Part model, mm, in its own coordinate system. Give positions to 0.01 mm unless a question says otherwise; leave off trailing zeros. Write each loop counter-clockwise with the first axis right and the second up, starting at its lowest first coordinate (ties: lowest second). Pieces come first, ordered by that corner, then holes. Notation, with made-up numbers: M 36,27 L 91,27 A17 ccw 91,33 Z; hole C 61,-30 d1. An arc over 180 degrees is marked long. Answer as CSV lines item,"result". Start each with the question number.
Item 1: Pin check, flat tips, straight feed: pin 1 (3 mm diameter, centred on x = 26.55, z = 20.3, fed in from -Y) (3 decimals); pin 2 (1.9 mm diameter, centred on y = 4.5, z = -43.5, fed in from -X). Stop position of each tip, or through.
Item 2: Band-saw the part on B-B, the plane y = 3.25. Count the separate pieces of the cut face and the enclosed holes in it, then the cut area to 3 significant figures.
Item 3: Band-saw the part on A-A, the plane x = 0. List the corners of the cut face in (y, z), then the cut area to 3 significant figures.
Item 4: Wall check: L1, parallel to X at y = 2, z = 0; L2, parallel to Z at x = 0, y = 3.5; L3, parallel to Z at x = 46.5, y = 2.75. Give the ranges that are in metal, low to high. Write a range as from..to.
from build123d import *

# Parameters (mm, degrees)
SKETCH2_W           = 154.686
SKETCH2_H           = 228.6
BOSS_EXTRUDE1_DEPTH = 6.35
SKETCH1_R           = 2.2225
CUT_EXTRUDE1_DEPTH  = 6.35
SKETCH3_W           = 15.24
SKETCH3_H           = 50.8
CUT_EXTRUDE2_DEPTH  = 6.35
SKETCH8_R           = 2.54
CUT_EXTRUDE3_DEPTH  = 17.78
SKETCH10_R          = 2
CUT_EXTRUDE4_DEPTH  = 7.35


with BuildPart() as part:
    # Sketch2 → Boss-Extrude1 (new body)
    with BuildSketch(Plane(origin=(0, 0, 0), x_dir=(1, 0, 0), z_dir=(0, 1, 0))):
        with Locations((26.543, 26.944051327)):
            Rectangle(SKETCH2_W, SKETCH2_H)
    extrude(amount=BOSS_EXTRUDE1_DEPTH)

    # Sketch1 → Cut-Extrude1 (cut)
    with BuildSketch(Plane(origin=(0, 0, 0), x_dir=(1, 0, 0), z_dir=(0, 1, 0))):
        with Locations((0, 90.444051327)):
            Circle(SKETCH1_R)
        with Locations((53.086, 90.444051327)):
            Circle(SKETCH1_R)
        Circle(SKETCH1_R)
        with Locations((53.086, 0)):
            Circle(SKETCH1_R)
    extrude(amount=CUT_EXTRUDE1_DEPTH, mode=Mode.SUBTRACT)

    # Sketch3 → Cut-Extrude2 (cut)
    with BuildSketch(Plane(origin=(0, 6.35, 0), x_dir=(1, 0, 0), z_dir=(0, 1, 0))):
        with Locations((96.266, 56.154051327)):
            Rectangle(SKETCH3_W, SKETCH3_H)
        with Locations((-43.18, 56.154051327)):
            Rectangle(SKETCH3_W, SKETCH3_H)
    extrude(amount=-CUT_EXTRUDE2_DEPTH, mode=Mode.SUBTRACT)

    # Sketch8 → Cut-Extrude3 (cut)
    with BuildSketch(Plane(origin=(0, 6.35, 0), x_dir=(1, 0, 0), z_dir=(0, 1, 0))):
        with Locations((26.550112, -20.29968)):
            Circle(SKETCH8_R)
        with Locations((-23.077082804, 0.02032)):
            Circle(SKETCH8_R)
        with Locations((76.177306804, 0.02032)):
            Circle(SKETCH8_R)
    extrude(amount=-CUT_EXTRUDE3_DEPTH, mode=Mode.SUBTRACT)

    # Sketch10 → Cut-Extrude4 (cut, through all)
    with BuildSketch(Plane(origin=(0, 6.35, 0), x_dir=(1, 0, 0), z_dir=(0, 1, 0))):
        with Locations((6.604, 7.005051327)):
            Circle(SKETCH10_R)
        with Locations((46.482, 7.005051327)):
            Circle(SKETCH10_R)
        with Locations((46.482, 46.883051327)):
            Circle(SKETCH10_R)
        with Locations((6.604, 46.883051327)):
            Circle(SKETCH10_R)
    extrude(amount=-CUT_EXTRUDE4_DEPTH, mode=Mode.SUBTRACT)


solid = part.part
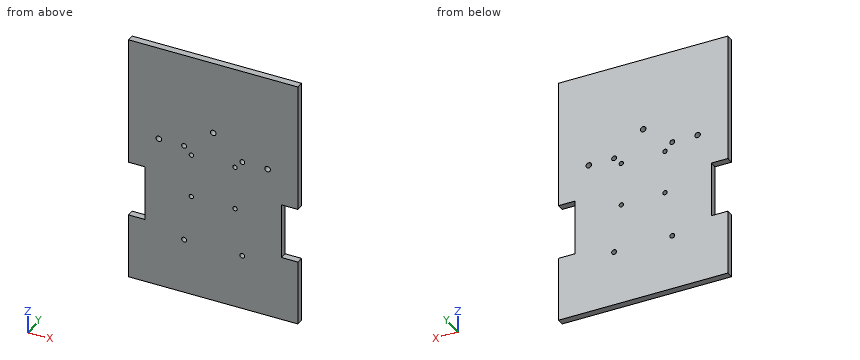
Output:
1,pin 1,"through"
1,pin 2,"x = -35.56"
2,separate pieces,"1"
2,enclosed holes,"11"
2,area,"33,600 mm²"
3,outline,"M 0,-141.24 L 6.35,-141.24 L 6.35,-92.67 L 0,-92.67 Z; M 0,-88.22 L 6.35,-88.22 L 6.35,-2.22 L 0,-2.22 Z; M 0,2.22 L 6.35,2.22 L 6.35,87.36 L 0,87.36 Z"
3,area,"1,400 mm²"
4,L1,"-50.8..-25.62, -20.54..-2.22, 2.22..50.86, 55.31..73.64, 78.72..103.89"
4,L2,"-141.24..-92.67, -88.22..-2.22, 2.22..87.36"
4,L3,"-141.24..-48.88, -44.88..-9, -5.01..87.36"
